For this review, take the finished solid that the model builds, in its own axes (mm). A direction names the side the tool comes from. Round coordinates to 2 decimals unless told otherwise and drop trailing zeros. Order: outer loops, then holes, each group sorted by start corner. A loop starts at its lowest first (then second) coordinate and runs counter-clockwise, first axis right, second up. Notation, with made-up numbers: (-17, -33.75) - (-10, -33.75) arc R20 ccw to (-10, -23.75) - close; hole circle Ø5 at (-29.75, -20). An arc over 180 degrees is marked (long way). One line per item, written item: value.
```python
from build123d import *

# Parameters (mm, degrees)
SKETCH2_W           = 170
SKETCH2_H           = 100
BOSS_EXTRUDE5_DEPTH = 154
SHELL1_T            = -3
SKETCH6_W           = 94
SKETCH6_H           = 30.059246991
BOSS_EXTRUDE6_DEPTH = 55
SKETCH7_W           = 78
SKETCH7_H           = 30.059246991
CUT_EXTRUDE3_DEPTH  = 55
SKETCH8_R           = 6.925
CUT_EXTRUDE5_DEPTH  = 94
FILLET1_R           = 10
CUT_EXTRUDE6_REACH  = 216.047
SKETCH9_R           = 42.5


with BuildPart() as part:
    # Sketch2 → Boss-Extrude5 (new body)
    with BuildSketch(Plane(origin=(0, 0, 0), x_dir=(0, 0, -1), z_dir=(1, 0, 0))):
        Rectangle(SKETCH2_W, SKETCH2_H)
    extrude(amount=BOSS_EXTRUDE5_DEPTH)

    # Shell1
    shell1_openings = [part.faces().sort_by_distance(p)[0] for p in [
        (77, 50, 0),
    ]]
    offset(amount=SHELL1_T, openings=shell1_openings, kind=Kind.INTERSECTION)

    # Sketch6 → Boss-Extrude6 (add)
    with BuildSketch(Plane.XY.offset(85)):
        with Locations((77, -34.970376505)):
            Rectangle(SKETCH6_W, SKETCH6_H)
    extrude(amount=BOSS_EXTRUDE6_DEPTH)

    # Sketch7 → Cut-Extrude3 (cut)
    with BuildSketch(Plane.XY.offset(140)):
        with Locations((77, -34.970376505)):
            Rectangle(SKETCH7_W, SKETCH7_H)
    extrude(amount=-CUT_EXTRUDE3_DEPTH, mode=Mode.SUBTRACT)

    # Sketch8 → Cut-Extrude5 (cut)
    with BuildSketch(Plane(origin=(124, 0, 0), x_dir=(0, 0, -1), z_dir=(1, 0, 0))):
        with Locations((-127.5, -34.970376505)):
            Circle(SKETCH8_R)
    extrude(amount=-CUT_EXTRUDE5_DEPTH, mode=Mode.SUBTRACT)

    # Fillet1
    fillet1_edges = [part.edges().sort_by_distance(p)[0] for p in [
        (34, -19.940753009, 140),
        (34, -50, 140),
        (120, -50, 140),
        (120, -19.940753009, 140),
    ]]
    fillet(fillet1_edges, radius=FILLET1_R)

    # Cut-Extrude6: up to this face of the body (flat: up to its plane)
    cut_extrude6_end = Plane(part.part.faces().sort_by_distance((0, 0, 0))[0])
    # Sketch9 → Cut-Extrude6 (cut, up to the picked face)
    with BuildSketch(Plane(origin=(154, 0, 0), x_dir=(0, 0, -1), z_dir=(1, 0, 0)), mode=Mode.PRIVATE) as cut_extrude6_sk1:
        with Locations((85, 50)):
            Circle(SKETCH9_R)
    cut_extrude6_tool1 = split(extrude(cut_extrude6_sk1.sketch, amount=-CUT_EXTRUDE6_REACH, mode=Mode.PRIVATE), bisect_by=cut_extrude6_end, keep=Keep.BOTH, mode=Mode.PRIVATE)
    # Sketch9 → Cut-Extrude6 (cut, up to the picked face)
    with BuildSketch(Plane(origin=(154, 0, 0), x_dir=(0, 0, -1), z_dir=(1, 0, 0)), mode=Mode.PRIVATE) as cut_extrude6_sk2:
        with Locations((-85, 50)):
            Circle(SKETCH9_R)
    cut_extrude6_tool2 = split(extrude(cut_extrude6_sk2.sketch, amount=-CUT_EXTRUDE6_REACH, mode=Mode.PRIVATE), bisect_by=cut_extrude6_end, keep=Keep.BOTH, mode=Mode.PRIVATE)
    add(cut_extrude6_tool1.solids().sort_by(Axis((154, 50, -85), (-1, 0, 0)))[0], mode=Mode.SUBTRACT)
    add(cut_extrude6_tool2.solids().sort_by(Axis((154, 50, 85), (-1, 0, 0)))[0], mode=Mode.SUBTRACT)


solid = part.part
```
Item 1: For P1, Ø15, axis at y = -29, z = 109.5, coming from the +X side; P2, Ø9, axis at y = -29, z = 100.5, coming from the -X side; P3, Ø2.5, axis at x = 120.5, z = 105.5, coming from the +Y side; P4, Ø11, axis at y = -34.97, z = 127.5, coming from the +X side, all flat-tipped, find the tip position at first contact; note any pin that passes through.
Returned:
P1: x = 124
P2: x = 30
P3: y = -19.94
P4: through
Item 2: Machinability: for faces 1 (the flat face through (76, -20, 82)), 2 (the flat face through (124, -35, 112)), 3 (the flat face through (120, -19.941, 107)), which of the approach directions +Z, -Z, +X, -X, +Y, -Y give a long, thin tool a straight path to every point of the face, cutting with its end or side? Answer none if there is none.
Returned:
face 1: +Y
face 2: +Z, +X, +Y, -Y
face 3: +Z, +X, -X, +Y
Item 3: Take a section at C-C (x = 33). Write out the cut boundary in (y, z) (3 decimals), plus the area to 3 significant figures.
Returned:
outline: (-50, -85) - (7.5, -85) arc R42.5 cw to (7.606, -82) - (-47, -82) - (-47, 82) - (7.606, 82) arc R42.5 cw to (7.5, 85) - (-19.941, 85) - (-19.941, 130) arc R10 ccw to (-29.941, 140) - (-40, 140) arc R10 ccw to (-50, 130) - close; hole circle Ø13.85 at (-34.97, 127.5)
area: 2,300 mm^2
Item 4: The part is to be moulded in two halves that separate along X. For faces 4 (the flat face through (154, -10, 1)), 5 (the flat face through (3, -9, 1)), 6 (the cylindrical face through (120.06, -47.15, 136.99)), say which applies: +X half, -X half, draft (parallel to the pull), parting line (faces both ways), or undercut.
Returned:
face 4: +X half
face 5: undercut
face 6: draft
Item 5: Take a section at D-D (y = 0). Write out the cut boundary in (x, z), plus the area to 3 significant figures.
Returned:
outline: (0, -85) - (154, -85) - (154, 85) - (0, 85) - close; hole (3, -82) - (151, -82) - (151, 82) - (3, 82) - close
area: 1,910 mm^2
Item 6: Take a section at A-A (z = 127.5). Write out the cut boundary in (x, y).
Returned:
outline: (30, -50) - (38, -50) - (38, -41.9) - (30, -41.9) - close; (30, -28.05) - (38, -28.05) - (38, -19.94) - (30, -19.94) - close; (116, -50) - (124, -50) - (124, -41.9) - (116, -41.9) - close; (116, -28.05) - (124, -28.05) - (124, -19.94) - (116, -19.94) - close
Item 7: Take a section at B-B (y = 10.5). Write out the cut boundary in (x, z).
Returned:
outline: (0, -69.32) - (3, -69.32) - (3, 69.32) - (0, 69.32) - close; (151, -69.32) - (154, -69.32) - (154, 69.32) - (151, 69.32) - close
Item 8: Wall thickness on line 1 (Z direction, x = 83, y = 2.5); line 2 (X direction, y = -44.5, z = 57); line 3 (Y direction, x = 118.75, z = 127.5): over which ranges is each line inside the solid? List them lowest first.
Returned:
line 1: -85 to -82, 82 to 85
line 2: 0 to 3, 151 to 154
line 3: -50 to -41.9, -28.05 to -19.94
